Geometry check sheet. Reference: the model listing, model coordinates, mm. A direction names the side the tool comes from. Coordinates: 2 decimals unless noted, no trailing zeros. Order: outer loops, then holes, each group sorted by start corner. A loop starts at its lowest first (then second) coordinate and runs counter-clockwise, first axis right, second up. Notation, with made-up numbers: (-26.5, -14.75) -> (22.5, -14.75) arc R19 cw to (22.5, 11.25) -> close; hole circle Ø1 at (-16, 67.25). An arc over 180 degrees is marked (long way). Answer in a Markdown table with one row per item. Add a question column.
```python
from build123d import *

# Parameters (mm, degrees)
F0_R     = 12.5
F1_DEPTH = 10


with BuildPart() as f1:
    # F0 (on Top) → F1 (new body)
    with BuildSketch(Plane.XY):
        with BuildLine():
            ThreePointArc((0, 17.5), (5.125631, 5.125631), (17.5, 0))
            Line((17.5, 0), (133, 0))
            ThreePointArc((133, 0), (136.535534, 1.464466), (138, 5))
            Line((138, 5), (138, 30))
            ThreePointArc((138, 30), (136.535534, 33.535534), (133, 35))
            Line((133, 35), (17.5, 35))
            ThreePointArc((17.5, 35), (5.125631, 29.874369), (0, 17.5))
        make_face()
        with Locations((17.5, 17.5)):
            Circle(F0_R, mode=Mode.SUBTRACT)
    extrude(amount=F1_DEPTH)

    # F2 (on face) → F3 (revolve, cut)
    with BuildSketch(Plane.XY.offset(10)):
        Polygon((44, 19), (44, 7), (48.5, 7), (48.5, 19), (53, 19), (53, 24), (51.5, 24), (51.5, 29), (44, 29), (44, 24), align=None)
    revolve(axis=Axis((44, 13, 10), (0, 1, 0)), mode=Mode.SUBTRACT)

    # F2 (on face) → F4 (revolve, cut)
    with BuildSketch(Plane.XY.offset(10)):
        Polygon((64, 19), (64, 7), (68.5, 7), (68.5, 19), (73, 19), (73, 24), (71.5, 24), (71.5, 29), (64, 29), (64, 24), align=None)
    revolve(axis=Axis((64, 21.5, 10), (0, 1, 0)), mode=Mode.SUBTRACT)

    # F2 (on face) → F5 (revolve, cut)
    with BuildSketch(Plane.XY.offset(10)):
        Polygon((84, 19), (84, 7), (88.5, 7), (88.5, 19), (93, 19), (93, 24), (91.5, 24), (91.5, 29), (84, 29), (84, 24), align=None)
    revolve(axis=Axis((84, 21.5, 10), (0, 1, 0)), mode=Mode.SUBTRACT)

    # F2 (on face) → F6 (revolve, cut)
    with BuildSketch(Plane.XY.offset(10)):
        Polygon((104, 19), (104, 7), (108.5, 7), (108.5, 19), (113, 19), (113, 24), (111.5, 24), (111.5, 29), (104, 29), (104, 24), align=None)
    revolve(axis=Axis((104, 13, 10), (0, 1, 0)), mode=Mode.SUBTRACT)

    # F2 (on face) → F7 (revolve, cut)
    with BuildSketch(Plane.XY.offset(10)):
        Polygon((124, 19), (124, 7), (128.5, 7), (128.5, 19), (133, 19), (133, 24), (131.5, 24), (131.5, 29), (124, 29), (124, 24), align=None)
    revolve(axis=Axis((124, 13, 10), (0, 1, 0)), mode=Mode.SUBTRACT)


solid = f1.part
```
(1) Cross-section at D-D (y = 3.5). Enter the section's corners in (x, z).
(2) Cross-section at C-C (y = 32.5). Enter the section's corners in (x, z).
(3) Cross-section at B-B (z = 4). Give the number of separate pieces and of enclosed holes in the cut face, plus the area to 3 significant figures.
(4) Scan lines: line 1 along Y through (x, z) = (17.5, 7.75); line 2 along Y through (x, z) = (104, 7.5); line 3 along X through (y, z) = (15, 0.5). Record each from-to range of solid material in increasing order.
(5) Access from +Z, -Z, +X, -X, +Y, -Y to the whole of each face (thin tool, end or side, straight path). Record for faces 4 (the face through (76, 35, 5)), 5 (the face through (44.16, 26.54, 2.5)).
(6) Mould release check, pull along Y, two halves, no side actions. Record for faces 1 (the face through (44, 19, 5)), 2 (the face through (136, 1, 5)), 3 (the face through (83, 18, 0)): +Y half, -Y half, draft (parallel to the pull), parting line (faces both ways), or undercut.
(7) Cross-section at A-A (x = 44). Enter the section's corners in (y, z), plus the area to 4 significant figures.
Checks:
| question | item | result |
|---|---|---|
| 1 | outline | (7, 0) -> (137.77, 0) -> (137.77, 10) -> (7, 10) -> close |
| 2 | outline | (8.49, 0) -> (137.33, 0) -> (137.33, 10) -> (8.49, 10) -> close |
| 3 | separate pieces | 1 |
| 3 | enclosed holes | 6 |
| 3 | area | 3,640 mm² |
| 4 | line 1 | 0 to 5, 30 to 35 |
| 4 | line 2 | 0 to 7, 29 to 35 |
| 4 | line 3 | 0.18 to 5.25, 29.75 to 138 |
| 5 | face 4 | +Z, -Z, +X, -X, +Y |
| 5 | face 5 | +Z |
| 6 | face 1 | undercut |
| 6 | face 2 | -Y half |
| 6 | face 3 | draft |
| 7 | outline | (0, 0) -> (35, 0) -> (35, 10) -> (29, 10) -> (29, 2.5) -> (24, 2.5) -> (24, 1) -> (19, 1) -> (19, 5.5) -> (7, 5.5) -> (7, 10) -> (0, 10) -> close |
| 7 | area | 213.5 mm² |
